Input: part model. Units: mm. Frame: model coordinates. Coordinates: 2 decimals unless noted, no trailing zeros. Write each loop counter-clockwise with the first axis right and the second up, starting at its lowest first coordinate (ties: lowest second). Pieces come first, ordered by that corner, then holes.
from build123d import *

# Parameters (mm, degrees)
SKETCH1_W           = 436
SKETCH1_H           = 112.5
BOSS_EXTRUDE1_DEPTH = 6
SKETCH2_W           = 22.5
SKETCH2_H           = 6
BOSS_EXTRUDE2_DEPTH = 6
SKETCH3_W           = 39.636363637
SKETCH3_H           = 6
SKETCH3_W_2         = 39.636363636
BOSS_EXTRUDE3_DEPTH = 6
SKETCH4_W           = 6
SKETCH4_H           = 22.5
CUT_EXTRUDE1_DEPTH  = 6
CUT_EXTRUDE2_DEPTH  = 7


with BuildPart() as part:
    # Sketch1 → Boss-Extrude1 (new body)
    with BuildSketch(Plane(origin=(0, 0, 0), x_dir=(1, 0, 0), z_dir=(0, 1, 0))):
        Rectangle(SKETCH1_W, SKETCH1_H)
    extrude(amount=BOSS_EXTRUDE1_DEPTH)

    # Sketch2 → Boss-Extrude2 (add)
    with BuildSketch(Plane.ZY.offset(218)):
        with Locations((-22.5, 3)):
            Rectangle(SKETCH2_W, SKETCH2_H)
        with Locations((22.5, 3)):
            Rectangle(SKETCH2_W, SKETCH2_H)
    boss_extrude2 = extrude(amount=BOSS_EXTRUDE2_DEPTH)

    # Mirror1: Boss-Extrude2 across plane
    add(boss_extrude2.mirror(Plane(origin=(0, 0, 0), x_dir=(0, 0, 1), z_dir=(1, 0, 0))))

    # Sketch3 → Boss-Extrude3 (add)
    with BuildSketch(Plane(origin=(0, 0, -56.25), x_dir=(-1, 0, 0), z_dir=(0, 0, -1))):
        with Locations((158.545454546, 3)):
            Rectangle(SKETCH3_W, SKETCH3_H)
        with Locations((79.272727273, 3)):
            Rectangle(SKETCH3_W_2, SKETCH3_H)
        with Locations((0, 3)):
            Rectangle(SKETCH3_W_2, SKETCH3_H)
        with Locations((-79.272727273, 3)):
            Rectangle(SKETCH3_W_2, SKETCH3_H)
        with Locations((-158.545454546, 3)):
            Rectangle(SKETCH3_W, SKETCH3_H)
    boss_extrude3 = extrude(amount=BOSS_EXTRUDE3_DEPTH)

    # Mirror2: Boss-Extrude3 across Front Plane
    add(boss_extrude3.mirror(Plane.XY))

    # Sketch4 → Cut-Extrude1 (cut)
    with BuildSketch(Plane.XZ):
        with Locations((191, 22.5)):
            Rectangle(SKETCH4_W, SKETCH4_H)
        with Locations((191, -22.5)):
            Rectangle(SKETCH4_W, SKETCH4_H)
    extrude(amount=-CUT_EXTRUDE1_DEPTH, mode=Mode.SUBTRACT)

    # Sketch5 → Cut-Extrude2 (cut, through all)
    with BuildSketch(Plane(origin=(0, 6, 0), x_dir=(1, 0, 0), z_dir=(0, 1, 0))):
        with BuildLine():
            Line((-54.8, 21.15), (-24.8, 21.15))
            ThreePointArc((-24.8, 21.15), (-23.9, 20.25), (-24.8, 19.35))
            Line((-24.8, 19.35), (-54.8, 19.35))
            ThreePointArc((-54.8, 19.35), (-55.7, 20.25), (-54.8, 21.15))
        make_face()
        with BuildLine():
            Line((-15, 21.15), (15, 21.15))
            ThreePointArc((15, 21.15), (15.9, 20.25), (15, 19.35))
            Line((15, 19.35), (-15, 19.35))
            ThreePointArc((-15, 19.35), (-15.9, 20.25), (-15, 21.15))
        make_face()
        with BuildLine():
            Line((54.8, 21.15), (24.8, 21.15))
            ThreePointArc((24.8, 21.15), (23.9, 20.25), (24.8, 19.35))
            Line((24.8, 19.35), (54.8, 19.35))
            ThreePointArc((54.8, 19.35), (55.7, 20.25), (54.8, 21.15))
        make_face()
        with BuildLine():
            Line((-54.8, 14.4), (-24.8, 14.4))
            ThreePointArc((-24.8, 14.4), (-23.9, 13.5), (-24.8, 12.6))
            Line((-24.8, 12.6), (-54.8, 12.6))
            ThreePointArc((-54.8, 12.6), (-55.7, 13.5), (-54.8, 14.4))
        make_face()
        with BuildLine():
            Line((-15, 14.4), (15, 14.4))
            ThreePointArc((15, 14.4), (15.9, 13.5), (15, 12.6))
            Line((15, 12.6), (-15, 12.6))
            ThreePointArc((-15, 12.6), (-15.9, 13.5), (-15, 14.4))
        make_face()
        with BuildLine():
            Line((54.8, 14.4), (24.8, 14.4))
            ThreePointArc((24.8, 14.4), (23.9, 13.5), (24.8, 12.6))
            Line((24.8, 12.6), (54.8, 12.6))
            ThreePointArc((54.8, 12.6), (55.7, 13.5), (54.8, 14.4))
        make_face()
        with BuildLine():
            Line((-54.8, 7.65), (-24.8, 7.65))
            ThreePointArc((-24.8, 7.65), (-23.9, 6.75), (-24.8, 5.85))
            Line((-24.8, 5.85), (-54.8, 5.85))
            ThreePointArc((-54.8, 5.85), (-55.7, 6.75), (-54.8, 7.65))
        make_face()
        with BuildLine():
            Line((-15, 7.65), (15, 7.65))
            ThreePointArc((15, 7.65), (15.9, 6.75), (15, 5.85))
            Line((15, 5.85), (-15, 5.85))
            ThreePointArc((-15, 5.85), (-15.9, 6.75), (-15, 7.65))
        make_face()
        with BuildLine():
            Line((54.8, 7.65), (24.8, 7.65))
            ThreePointArc((24.8, 7.65), (23.9, 6.75), (24.8, 5.85))
            Line((24.8, 5.85), (54.8, 5.85))
            ThreePointArc((54.8, 5.85), (55.7, 6.75), (54.8, 7.65))
        make_face()
        with BuildLine():
            Line((-54.8, 0.9), (-24.8, 0.9))
            ThreePointArc((-24.8, 0.9), (-23.9, 0), (-24.8, -0.9))
            Line((-24.8, -0.9), (-54.8, -0.9))
            ThreePointArc((-54.8, -0.9), (-55.7, 0), (-54.8, 0.9))
        make_face()
        with BuildLine():
            Line((-15, 0.9), (15, 0.9))
            ThreePointArc((15, 0.9), (15.9, 0), (15, -0.9))
            Line((15, -0.9), (-15, -0.9))
            ThreePointArc((-15, -0.9), (-15.9, 0), (-15, 0.9))
        make_face()
        with BuildLine():
            Line((54.8, 0.9), (24.8, 0.9))
            ThreePointArc((24.8, 0.9), (23.9, 0), (24.8, -0.9))
            Line((24.8, -0.9), (54.8, -0.9))
            ThreePointArc((54.8, -0.9), (55.7, 0), (54.8, 0.9))
        make_face()
        with BuildLine():
            Line((-54.8, -5.85), (-24.8, -5.85))
            ThreePointArc((-24.8, -5.85), (-23.9, -6.75), (-24.8, -7.65))
            Line((-24.8, -7.65), (-54.8, -7.65))
            ThreePointArc((-54.8, -7.65), (-55.7, -6.75), (-54.8, -5.85))
        make_face()
        with BuildLine():
            Line((-15, -5.85), (15, -5.85))
            ThreePointArc((15, -5.85), (15.9, -6.75), (15, -7.65))
            Line((15, -7.65), (-15, -7.65))
            ThreePointArc((-15, -7.65), (-15.9, -6.75), (-15, -5.85))
        make_face()
        with BuildLine():
            Line((54.8, -5.85), (24.8, -5.85))
            ThreePointArc((24.8, -5.85), (23.9, -6.75), (24.8, -7.65))
            Line((24.8, -7.65), (54.8, -7.65))
            ThreePointArc((54.8, -7.65), (55.7, -6.75), (54.8, -5.85))
        make_face()
        with BuildLine():
            Line((-54.8, -12.6), (-24.8, -12.6))
            ThreePointArc((-24.8, -12.6), (-23.9, -13.5), (-24.8, -14.4))
            Line((-24.8, -14.4), (-54.8, -14.4))
            ThreePointArc((-54.8, -14.4), (-55.7, -13.5), (-54.8, -12.6))
        make_face()
        with BuildLine():
            Line((-15, -12.6), (15, -12.6))
            ThreePointArc((15, -12.6), (15.9, -13.5), (15, -14.4))
            Line((15, -14.4), (-15, -14.4))
            ThreePointArc((-15, -14.4), (-15.9, -13.5), (-15, -12.6))
        make_face()
        with BuildLine():
            Line((54.8, -12.6), (24.8, -12.6))
            ThreePointArc((24.8, -12.6), (23.9, -13.5), (24.8, -14.4))
            Line((24.8, -14.4), (54.8, -14.4))
            ThreePointArc((54.8, -14.4), (55.7, -13.5), (54.8, -12.6))
        make_face()
        with BuildLine():
            Line((-54.8, -19.35), (-24.8, -19.35))
            ThreePointArc((-24.8, -19.35), (-23.9, -20.25), (-24.8, -21.15))
            Line((-24.8, -21.15), (-54.8, -21.15))
            ThreePointArc((-54.8, -21.15), (-55.7, -20.25), (-54.8, -19.35))
        make_face()
        with BuildLine():
            Line((-15, -19.35), (15, -19.35))
            ThreePointArc((15, -19.35), (15.9, -20.25), (15, -21.15))
            Line((15, -21.15), (-15, -21.15))
            ThreePointArc((-15, -21.15), (-15.9, -20.25), (-15, -19.35))
        make_face()
        with BuildLine():
            Line((54.8, -19.35), (24.8, -19.35))
            ThreePointArc((24.8, -19.35), (23.9, -20.25), (24.8, -21.15))
            Line((24.8, -21.15), (54.8, -21.15))
            ThreePointArc((54.8, -21.15), (55.7, -20.25), (54.8, -19.35))
        make_face()
    extrude(amount=-CUT_EXTRUDE2_DEPTH, mode=Mode.SUBTRACT)


solid = part.part
Item 1: Material intervals for line 1 (Z direction, x = 193.5, y = 2.8); line 2 (X direction, y = 0.6, z = 16.5); line 3 (X direction, y = 4.8, z = 13.5), sorted ascending.
Item 2: Pin query (flat end, axial travel): pin 1 Ø3 at (x, y) = (35, 2.5) entering from -Z; pin 2 Ø3 at (y, z) = (2, -60.5) entering from +X. Return the tip coordinate at first contact, or that it passes through.
Item 3: Section query C-C, the plane z = 50. Return loops of the section in (x, y).
Item 4: Section query D-D, the plane x = 132.5. Return loops of the section in (y, z).
Item 5: Section query A-A, the plane x = 34. State how many separate pieces and enclosed holes the cut face has, then the cut area to 3 significant figures.
The answers:
1. line 1: z = -56.25 to -33.75, -11.25 to 11.25, 33.75 to 56.25
1. line 2: x = -224 to 188, 194 to 224
1. line 3: x = -224 to -55.7, -23.9 to -15.9, 15.9 to 23.9, 55.7 to 188, 194 to 224
2. pin 1: stops at z = -56.25
2. pin 2: stops at x = 178.36
3. outline: (-218, 0) - (218, 0) - (218, 6) - (-218, 6) - close
4. outline: (0, -56.25) - (6, -56.25) - (6, 56.25) - (0, 56.25) - close
5. separate pieces: 8
5. enclosed holes: 0
5. area: 599 mm2
